CAD build for the part. Positions are in the model's coordinates, mm. A direction names the side the tool comes from. Round coordinates to 2 decimals unless told otherwise and drop trailing zeros. Loops run counter-clockwise (first coordinate to the right, second up) from the corner with the lowest first, then second, coordinate; pieces in that order, holes last.
from build123d import *

# Parameters (mm, degrees)
BOSS_EXTRUDE1_DEPTH = 3


with BuildPart() as part:
    # Sketch2 → Boss-Extrude1 (new body)
    with BuildSketch(Plane.XY):
        with BuildLine():
            ThreePointArc((13.72796065, -3.112181063), (12.035436414, 2.462021021), (16.770370099, 5.855657737))
            Line((16.770370099, 5.855657737), (46.770370099, 5.855657737))
            ThreePointArc((46.770370099, 5.855657737), (51.770370099, 0.855657737), (46.770370099, -4.144342263))
            Line((46.770370099, -4.144342263), (24.407279181, -4.144342263))
            ThreePointArc((24.407279181, -4.144342263), (24.217881833, -4.280087732), (24.285582803, -4.503055815))
            Line((24.285582803, -4.503055815), (26.943586158, -6.541126143))
            ThreePointArc((26.943586158, -6.541126143), (27.087190775, -6.617835631), (27.247827103, -6.644342263))
            Line((27.247827103, -6.644342263), (46.770370099, -6.644342263))
            ThreePointArc((46.770370099, -6.644342263), (54.270370099, 0.855657737), (46.770370099, 8.355657737))
            Line((46.770370099, 8.355657737), (1.770370099, 8.355657737))
            ThreePointArc((1.770370099, 8.355657737), (-5.729629901, 0.855657737), (1.770370099, -6.644342263))
            Line((1.770370099, -6.644342263), (17.747827103, -6.644342263))
            ThreePointArc((17.747827103, -6.644342263), (17.93260301, -6.520878949), (17.889248459, -6.302920907))
            Line((17.889248459, -6.302920907), (13.72796065, -3.112181063))
        make_face()
        with BuildLine():
            ThreePointArc((5.103723485, 3.20079905), (5.270370099, 3.120917237), (5.437016713, 3.20079905))
            ThreePointArc((5.437016713, 3.20079905), (5.635523651, 3.278293261), (5.802369663, 3.145730953))
            ThreePointArc((5.802369663, 3.145730953), (5.938067058, 3.020278113), (6.120855608, 3.047491049))
            ThreePointArc((6.120855608, 3.047491049), (6.33338526, 3.063031463), (6.453745345, 2.887179801))
            ThreePointArc((6.453745345, 2.887179801), (6.546436212, 2.727302969), (6.729125133, 2.699429041))
            ThreePointArc((6.729125133, 2.699429041), (6.936793306, 2.651634823), (6.999972944, 2.448118998))
            ThreePointArc((6.999972944, 2.448118998), (7.041421292, 2.268023934), (7.207777872, 2.18753986))
            ThreePointArc((7.207777872, 2.18753986), (7.392132338, 2.080657737), (7.392517739, 1.867561025))
            ThreePointArc((7.392517739, 1.867561025), (7.379040701, 1.683249963), (7.514283428, 1.557307108))
            ThreePointArc((7.514283428, 1.557307108), (7.658943484, 1.400834025), (7.596500404, 1.197091003))
            ThreePointArc((7.596500404, 1.197091003), (7.529295473, 1.024940791), (7.621407438, 0.864729731))
            ThreePointArc((7.621407438, 0.864729731), (7.713519402, 0.672569008), (7.593796183, 0.496283137))
            ThreePointArc((7.593796183, 0.496283137), (7.478834813, 0.351590078), (7.519631462, 0.171346267))
            ThreePointArc((7.519631462, 0.171346267), (7.551010783, -0.039427773), (7.384645358, -0.172592718))
            ThreePointArc((7.384645358, -0.172592718), (7.232142372, -0.276972013), (7.217998744, -0.46123312))
            ThreePointArc((7.217998744, -0.46123312), (7.185857231, -0.671892277), (6.987631898, -0.750104008))
            ThreePointArc((6.987631898, -0.750104008), (6.811137854, -0.804894979), (6.743310674, -0.976800975))
            ThreePointArc((6.743310674, -0.976800975), (6.650504241, -1.16862726), (6.438032191, -1.18493632))
            ThreePointArc((6.438032191, -1.18493632), (6.253229361, -1.18527055), (6.137745369, -1.329546832))
            ThreePointArc((6.137745369, -1.329546832), (5.992520276, -1.485495637), (5.784680583, -1.438452896))
            ThreePointArc((5.784680583, -1.438452896), (5.607989508, -1.384300685), (5.455109966, -1.488127674))
            ThreePointArc((5.455109966, -1.488127674), (5.270370099, -1.594342263), (5.085630232, -1.488127674))
            ThreePointArc((5.085630232, -1.488127674), (4.93275069, -1.384300685), (4.756059614, -1.438452896))
            ThreePointArc((4.756059614, -1.438452896), (4.548219922, -1.485495637), (4.402994828, -1.329546832))
            ThreePointArc((4.402994828, -1.329546832), (4.287510837, -1.18527055), (4.102708006, -1.18493632))
            ThreePointArc((4.102708006, -1.18493632), (3.890235957, -1.16862726), (3.797429524, -0.976800975))
            ThreePointArc((3.797429524, -0.976800975), (3.729602343, -0.804894979), (3.5531083, -0.750104008))
            ThreePointArc((3.5531083, -0.750104008), (3.354882967, -0.671892277), (3.322741454, -0.46123312))
            ThreePointArc((3.322741454, -0.46123312), (3.308597826, -0.276972013), (3.15609484, -0.172592718))
            ThreePointArc((3.15609484, -0.172592718), (2.989729415, -0.039427773), (3.021108735, 0.171346267))
            ThreePointArc((3.021108735, 0.171346267), (3.061905384, 0.351590078), (2.946944015, 0.496283137))
            ThreePointArc((2.946944015, 0.496283137), (2.827220796, 0.672569008), (2.91933276, 0.864729731))
            ThreePointArc((2.91933276, 0.864729731), (3.011444724, 1.024940791), (2.944239794, 1.197091003))
            ThreePointArc((2.944239794, 1.197091003), (2.881796714, 1.400834025), (3.02645677, 1.557307108))
            ThreePointArc((3.02645677, 1.557307108), (3.161699497, 1.683249963), (3.148222459, 1.867561025))
            ThreePointArc((3.148222459, 1.867561025), (3.14860786, 2.080657737), (3.332962326, 2.18753986))
            ThreePointArc((3.332962326, 2.18753986), (3.499318906, 2.268023934), (3.540767254, 2.448118998))
            ThreePointArc((3.540767254, 2.448118998), (3.603946891, 2.651634823), (3.811615065, 2.699429041))
            ThreePointArc((3.811615065, 2.699429041), (3.994303986, 2.727302969), (4.086994852, 2.887179801))
            ThreePointArc((4.086994852, 2.887179801), (4.207354938, 3.063031463), (4.41988459, 3.047491049))
            ThreePointArc((4.41988459, 3.047491049), (4.60267314, 3.020278113), (4.738370535, 3.145730953))
            ThreePointArc((4.738370535, 3.145730953), (4.905216547, 3.278293261), (5.103723485, 3.20079905))
        make_face(mode=Mode.SUBTRACT)
    extrude(amount=BOSS_EXTRUDE1_DEPTH)


solid = part.part
Item 1: Cut at B-B (y = -2.25). List the corners of the cut face in (x, z).
Verdict:
outline: (-5.06, 0) - (12.85, 0) - (12.85, 3) - (-5.06, 3) - close; (50.69, 0) - (53.6, 0) - (53.6, 3) - (50.69, 3) - close
Item 2: Mould opens along Y. For faces 1 (the cylindrical face through (-5.728, 1.021, 1.479)), 2 (the flat face through (15.8, -4.7, 1.5)), 3 (the flat face through (25.6, -5.51, 1.48)) say: released by +Y, released by -Y, zero draft, split by the parting line, or undercut.
Verdict:
face 1: split by the parting line
face 2: undercut
face 3: released by -Y
Item 3: Wall check: L1, parallel to Y at x = 44.5, z = 0.8; L2, parallel to X at y = -0.25, z = 0.95; L3, parallel to X at y = -1, z = 2.3. Give the ranges that are in metal, low to high.
Verdict:
L1: y = -6.64 to -4.14, 5.86 to 8.36
L2: x = -5.65 to 3.29, 7.25 to 11.89, 51.65 to 54.19
L3: x = -5.5 to 3.8, 6.74 to 12.13, 51.41 to 54.04
Item 4: 3-axis set-ups, long thin cutter, end or side, ignore diameter. For faces 4 (the cylindrical face through (12.01, 2.38, 1.48)), 5 (the flat face through (10, -6.644, 1)): which of +Z, -Z, +X, -X, +Y, -Y reach the whole face in a straight line?
Verdict:
face 4: +Z, -Z
face 5: +Z, -Z, +X, -X, -Y
Item 5: Flat gauge pin, fed straight in: P1, Ø1.5, axis at y = 2.5, z = 2, coming from the +X side. Where does the tip first touch, or does it go through?
Verdict:
P1: stops at x = 54.22
Item 6: Cut at A-A (x = 39). List the corners of the cut face in (y, z).
Verdict:
outline: (-6.64, 0) - (-4.14, 0) - (-4.14, 3) - (-6.64, 3) - close; (5.86, 0) - (8.36, 0) - (8.36, 3) - (5.86, 3) - close
